```python
from build123d import *

# Parameters (mm, degrees)
SKETCH1_R                = 3.025
BOSS_EXTRUDE1_DEPTH      = 4
BOSS_EXTRUDE2_DEPTH      = 3
BOSS_EXTRUDE2_DEPTH_BACK = 0.01
SKETCH2_R                = 7.5
BOSS_EXTRUDE3_DEPTH      = 2.5
CUT_EXTRUDE1_DEPTH       = 15.882876066
CUT_EXTRUDE1_DEPTH_BACK  = 15.882876066
SKETCH4_R                = 1


with BuildPart() as part:
    # Sketch1 → Boss-Extrude1 (new body)
    with BuildSketch(Plane(origin=(0, 0, 0), x_dir=(1, 0, 0), z_dir=(0, 1, 0))):
        with BuildLine():
            ThreePointArc((-4.431634889, 0.7814168), (-5.022292475, 3.232318908), (-4.820907073, 5.745333323))
            Line((-4.820907073, 5.745333323), (-2.892544244, 3.447199994))
            ThreePointArc((-2.892544244, 3.447199994), (-1.769604698, 5.704367313), (0, 7.5))
            Line((0, 7.5), (0, 4.5))
            ThreePointArc((0, 4.5), (2.311100785, 5.507278856), (4.820907073, 5.745333323))
            Line((4.820907073, 5.745333323), (2.892544244, 3.447199994))
            ThreePointArc((2.892544244, 3.447199994), (5.310416525, 2.733273415), (7.386058148, 1.302361333))
            Line((7.386058148, 1.302361333), (4.431634889, 0.7814168))
            ThreePointArc((4.431634889, 0.7814168), (5.824929355, -1.319661034), (6.495190528, -3.75))
            Line((6.495190528, -3.75), (3.897114317, -2.25))
            ThreePointArc((3.897114317, -2.25), (3.613893002, -4.755111418), (2.565151075, -7.047694656))
            Line((2.565151075, -7.047694656), (1.539090645, -4.228616794))
            ThreePointArc((1.539090645, -4.228616794), (-0.28812405, -5.965592323), (-2.565151075, -7.047694656))
            Line((-2.565151075, -7.047694656), (-1.539090645, -4.228616794))
            ThreePointArc((-1.539090645, -4.228616794), (-4.055324657, -4.384706279), (-6.495190528, -3.75))
            Line((-6.495190528, -3.75), (-3.897114317, -2.25))
            ThreePointArc((-3.897114317, -2.25), (-5.924993787, -0.752167437), (-7.386058148, 1.302361333))
            Line((-7.386058148, 1.302361333), (-4.431634889, 0.7814168))
        make_face()
        with Locations(Location((0, 0, 0), (0, 0, 270))):
            Circle(SKETCH1_R, mode=Mode.SUBTRACT)
    extrude(amount=BOSS_EXTRUDE1_DEPTH)

    # Sketch2 → Boss-Extrude2 (add, two sides: drawn at the far end of the back side and taken through both)
    with BuildSketch(Plane(origin=(0, 4, 0), x_dir=(1, 0, 0), z_dir=(0, 1, 0)).offset(-BOSS_EXTRUDE2_DEPTH_BACK)):
        with Locations(Location((0, 0, 0), (0, 0, 270))):
            Circle(SKETCH2_R)
    extrude(amount=BOSS_EXTRUDE2_DEPTH + BOSS_EXTRUDE2_DEPTH_BACK)

    # Sketch3 → Boss-Extrude3 (add)
    with BuildSketch(Plane(origin=(0, 7, 0), x_dir=(1, 0, 0), z_dir=(0, 1, 0))):
        Polygon((4.330127019, 7.5), (-4.330127019, 7.5), (-8.660254038, 0), (-4.330127019, -7.5), (4.330127019, -7.5), (8.660254038, 0), align=None)
    extrude(amount=BOSS_EXTRUDE3_DEPTH)

    # Sketch4 → Cut-Extrude1 (cut, two sides: drawn at the far end of the back side and taken through both)
    with BuildSketch(Plane(origin=(0, 0, 0), x_dir=(0, 0, -1), z_dir=(1, 0, 0)).offset(-CUT_EXTRUDE1_DEPTH_BACK)):
        with Locations((0, 5.49)):
            Circle(SKETCH4_R)
    extrude(amount=CUT_EXTRUDE1_DEPTH + CUT_EXTRUDE1_DEPTH_BACK, mode=Mode.SUBTRACT)

    # Cut-Sweep1: sweep along a path in Sketch2_2
    with BuildLine(Plane(origin=(0, 4, 0), x_dir=(1, 0, 0), z_dir=(0, 1, 0))) as cut_sweep1_path:
        CenterArc((0, 0), 7.5, 0, 360)
    # Sketch5 → Cut-Sweep1 (sweep, cut)
    with BuildSketch(Plane(origin=(0, 0, 0), x_dir=(0, 0, -1), z_dir=(1, 0, 0))):
        with BuildLine():
            Line((7.5, 7), (7.5, 3.99))
            ThreePointArc((7.5, 3.99), (7.095183038, 5.495), (7.5, 7))
        make_face()
    sweep(path=cut_sweep1_path.line, mode=Mode.SUBTRACT)


solid = part.part
```
Build history of the part. All positions in model axes, mm. A direction names the side the tool comes from. Round coordinates to 2 decimals unless told otherwise and drop trailing zeros. Write each loop counter-clockwise with the first axis right and the second up, starting at its lowest first coordinate (ties: lowest second). Pieces come first, ordered by that corner, then holes.
1) Drill centre lines: probe 1 along Y at (x, z) = (4, 0); probe 2 along Z at (x, y) = (3.75, 5.75); probe 3 along Y at (x, z) = (5, 5.75). Where is each one in solid material? Low to high.
2) Pin check, flat tips, straight feed: pin 1 (4 mm diameter, centred on x = -2, z = 6, fed in from -Y); pin 2 (3 mm diameter, centred on x = 0, z = -1, fed in from -Y); pin 3 (4 mm diameter, centred on y = 3.5, z = 2.5, fed in from -X); pin 4 (2 mm diameter, centred on x = 6.5, y = 1.5, fed in from -Z). Stop position of each tip, or through.
3) Band-saw the part on A-A, the plane y = 3. List the corners of the cut face in (x, z) (3 decimals).
4) 3-axis set-ups, long thin cutter, end or side, ignore diameter. For faces 5 (the flat face through (4, 7, -7)), 6 (the flat face through (3.87, 1.97, -4.61)), 7 (the flat face through (6.465, 8.232, 3.802)), 8 (the flat face through (-3, 3.99, -6)), 9 (the flat face through (-5.93, 1.967, -1.046)): which of +Z, -Z, +X, -X, +Y, -Y reach the whole face in a straight line?
5) Mould opens along X. For faces 1 (the flat face through (5.2, 2, 3)), 2 (the flat face through (5.93, 1.967, -1.046)), 3 (the flat face through (0, 9.5, 0)), 4 (the flat face through (-6.465, 8.232, -3.802)) say: +X half, -X half, draft (parallel to the pull), parting line (faces both ways), or undercut.
6) Band-saw the part on B-B, the plane y = 6. List the corners of the cut face in (x, z).
Ans:
1. probe 1: y = 0 to 4.49, 6.49 to 9.5
1. probe 2: z = -6.04 to -0.97, 0.97 to 6.04
1. probe 3: y = 7 to 9.5
2. pin 1: stops at y = 0
2. pin 2: stops at y = 3.99
2. pin 3: stops at x = -7.48
2. pin 4: stops at z = -2.64
3. outline: (-7.386, -1.302) - (-4.432, -0.781) arc R8 ccw to (-4.821, -5.745) - (-2.893, -3.447) arc R8 ccw to (0, -7.5) - (0, -4.5) arc R8 ccw to (4.821, -5.745) - (2.893, -3.447) arc R8 ccw to (7.386, -1.302) - (4.432, -0.781) arc R8 ccw to (6.495, 3.75) - (3.897, 2.25) arc R8 ccw to (2.565, 7.048) - (1.539, 4.229) arc R8 ccw to (-2.565, 7.048) - (-1.539, 4.229) arc R8 ccw to (-6.495, 3.75) - (-3.897, 2.25) arc R8 ccw to start; hole circle Ø6.05 at (0, 0)
4. face 5: -Z, +X, -Y
4. face 6: +X, -Y
4. face 7: +Z, +X, +Y, -Y
4. face 8: -Z, -Y
4. face 9: -Y
5. face 1: undercut
5. face 2: +X half
5. face 3: draft
5. face 4: -X half
6. outline: (-7.09, -0.86) arc R7.14 ccw to (7.09, -0.86) - close; (-7.09, 0.86) - (7.09, 0.86) arc R7.14 ccw to start
